```python
from build123d import *

# Parameters (mm, degrees)
SKETCH1_W           = 177.8
SKETCH1_H           = 101.6
BOSS_EXTRUDE1_DEPTH = 50.8
CUT_EXTRUDE1_DEPTH  = 178.8
BOSS_EXTRUDE2_DEPTH = 508


with BuildPart() as part:
    # Sketch1 → Boss-Extrude1 (new body)
    with BuildSketch(Plane(origin=(0, 0, 0), x_dir=(1, 0, 0), z_dir=(0, 1, 0))):
        with Locations((88.9, 50.8)):
            Rectangle(SKETCH1_W, SKETCH1_H)
    extrude(amount=BOSS_EXTRUDE1_DEPTH)

    # Sketch2 → Cut-Extrude1 (cut, through all)
    with BuildSketch(Plane(origin=(177.8, 0, 0), x_dir=(0, 0, -1), z_dir=(1, 0, 0))):
        Polygon((41.275, 0), (41.275, 6.858), (35.433, 12.7), (66.167, 12.7), (60.325, 6.858), (60.325, 0), align=None)
    extrude(amount=-CUT_EXTRUDE1_DEPTH, mode=Mode.SUBTRACT)

    # Sketch3 → Boss-Extrude2 (add)
    with BuildSketch(Plane(origin=(0, 50.8, 0), x_dir=(1, 0, 0), z_dir=(0, 1, 0))):
        Polygon((78.242626062, 31.429656714), (78.242626062, 38.287656714), (72.400626062, 44.129656714), (103.134626062, 44.129656714), (97.292626062, 38.287656714), (97.292626062, 31.429656714), align=None)
    extrude(amount=BOSS_EXTRUDE2_DEPTH)


solid = part.part
```
Source: CAD feature listing. Evaluate the final solid. Frame: model axes, mm. A direction names the side the tool comes from. Give positions to 0.01 mm unless a question says otherwise; leave off trailing zeros. Loops run counter-clockwise (first coordinate to the right, second up) from the corner with the lowest first, then second, coordinate; pieces in that order, holes last. Notation, with made-up numbers: (-39, -23) - (7, -23) arc R21 cw to (7, 16) - close; hole circle Ø1 at (-37.5, 21). An arc over 180 degrees is marked (long way). Use CSV: the item, a comma, the result in double quotes. Start each with the question number.
1. Section B-B (x = 48.5). Output: boundary loops of the cut face in (y, z) (3 decimals).
2. Reachability of faces 1 (the flat face through (88, 301, -31.43)), 2 (the flat face through (88, 301, -44.13)), 3 (the flat face through (88, 0, -81)) from +Z, -Z, +X, -X, +Y, -Y: full face, straight path, thin tool, end or side. Return the list, or none.
3. Section A-A (y = 455). Output: boundary loops of the cut face in (x, z).
4. Ray query, L1, parallel to Y at x = 121, z = -82; L2, parallel to X at y = 517, z = -37.5; L3, parallel to Y at x = 11.5, z = -43. Return the intervals inside material, ascending.
5. Pin query (flat end, axial travel): pin 1 (6 mm diameter, centred on y = 427, z = -30, fed in from +X); pin 2 (15 mm diameter, centred on x = 84.5, y = 399.5, fed in from +Z); pin 3 (2 mm diameter, centred on y = 375, z = -34, fed in from -X). Return the tip coordinate at first contact, or that it passes through.
6. Draft query along Y for faces 4 (the flat face through (90, 12.7, -51)), 5 (the flat face through (88, 0, -21)), 6 (the flat face through (88, 558.8, -39)). Return one class per face: +Y half, -Y half, draft (parallel to the pull), parting line (faces both ways), or undercut.
7. Section C-C (z = -19). Output: boundary loops of the cut face in (x, y).
Response:
1,outline,"(0, -101.6) - (50.8, -101.6) - (50.8, 0) - (0, 0) - (0, -41.275) - (6.858, -41.275) - (12.7, -35.433) - (12.7, -66.167) - (6.858, -60.325) - (0, -60.325) - close"
2,face 1,"+Z, +X, -X, +Y"
2,face 2,"-Z, +X, -X, +Y"
2,face 3,"+Z, -Z, +X, -X, -Y"
3,outline,"(72.4, -44.13) - (103.13, -44.13) - (97.29, -38.29) - (97.29, -31.43) - (78.24, -31.43) - (78.24, -38.29) - close"
4,L1,"0 to 50.8"
4,L2,"78.24 to 97.29"
4,L3,"12.7 to 50.8"
5,pin 1,"x = 97.29"
5,pin 2,"z = -31.43"
5,pin 3,"x = 78.24"
6,face 4,"undercut"
6,face 5,"-Y half"
6,face 6,"+Y half"
7,outline,"(0, 0) - (177.8, 0) - (177.8, 50.8) - (0, 50.8) - close"
